Geometry: final body of the model. Coordinates: model frame, mm. Coordinates: 2 decimals unless noted, no trailing zeros. Order: outer loops, then holes, each group sorted by start corner. A loop starts at its lowest first (then second) coordinate and runs counter-clockwise, first axis right, second up. Notation, with made-up numbers: M 47.5,58 L 57.5,58 A14 ccw 57.5,84 Z; hole C -39.5,82.5 d10. An arc over 180 degrees is marked long. Write item = value, one per line. Start each with the question number.
```python
from build123d import *

# Parameters (mm, degrees)
SKETCH_1_R                   = 100
SKETCH_1_R_2                 = 87
SKETCH_1_R_3                 = 2.25
EXTRUDE_1_DEPTH              = 8.5
HOLE_WIZARD_M4_1_D           = 4.8
HOLE_WIZARD_M4_1_CSINK_D     = 9.4
HOLE_WIZARD_M4_1_CSINK_ANGLE = 90


with BuildPart() as part:
    # ｽｹｯﾁ1 → ﾎﾞｽ - 押し出し1 (new body)
    with BuildSketch(Plane.XY):
        Circle(SKETCH_1_R)
        Circle(SKETCH_1_R_2, mode=Mode.SUBTRACT)
        with Locations((0, 93.5)):
            Circle(SKETCH_1_R_3, mode=Mode.SUBTRACT)
        with Locations((93.5, 0)):
            Circle(SKETCH_1_R_3, mode=Mode.SUBTRACT)
        with Locations((0, -93.5)):
            Circle(SKETCH_1_R_3, mode=Mode.SUBTRACT)
        with Locations((-93.5, 0)):
            Circle(SKETCH_1_R_3, mode=Mode.SUBTRACT)
    extrude(amount=EXTRUDE_1_DEPTH)

    # M4 丸皿ねじ用皿穴1 (through all)
    with Locations(Plane.XY.offset(8.5)):
        with Locations((-93.5, 0), (0, 93.5), (93.5, 0), (0, -93.5)):
            CounterSinkHole(HOLE_WIZARD_M4_1_D / 2, HOLE_WIZARD_M4_1_CSINK_D / 2, counter_sink_angle=HOLE_WIZARD_M4_1_CSINK_ANGLE)


solid = part.part
```
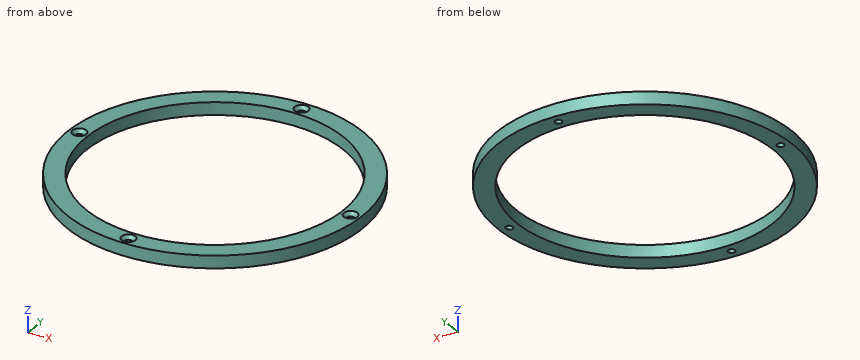
Item 1: Section query C-C on z = 1.75. Output: boundary loops of the cut face in (x, y), and give its area (3 significant figures).
Item 2: First-contact query: pin 1 (3 mm diameter, centred on x = 0, y = -93.5, fed in from -Z); pin 2 (1.5 mm diameter, centred on x = 7, z = 7.5, fed in from -Y); pin 3 (5 mm diameter, centred on y = -33.5, z = 5.5, fed in from -X); pin 4 (4 mm diameter, centred on x = 29, z = 1.5, fed in from -Y). Flat tips, straight axial feed; report the tip coordinate or a pass-through.
Item 3: Material intervals for probe 1 along Y at (x, z) = (0, 3.5); probe 2 along X at (y, z) = (50, 3); probe 3 along Y at (x, z) = (-32, 7.5), sorted ascending. Write a range as [from, to].
Item 4: Section query B-B on y = -60. Output: boundary loops of the cut face in (x, z).
Item 5: Section query A-A on x = 0. Output: boundary loops of the cut face in (y, z), and give its area (3 significant figures).
Ans:
q1.outline = C 0,0 d200; hole C -93.5,0 d4.8; hole C 0,0 d174; hole C 0,-93.5 d4.8; hole C 0,93.5 d4.8; hole C 93.5,0 d4.8
q1.area = 7,560 mm^2
q2.pin_1 = through
q2.pin_2 = -99.8
q2.pin_3 = -95.07
q2.pin_4 = -96.29
q3.probe_1 = [-100, -95.9], [-91.1, -87], [87, 91.1], [95.9, 100]
q3.probe_2 = [-86.6, -71.2], [71.2, 86.6]
q3.probe_3 = [-94.74, -80.9], [80.9, 94.74]
q4.outline = M -80,0 L -63,0 L -63,8.5 L -80,8.5 Z; M 63,0 L 80,0 L 80,8.5 L 63,8.5 Z
q5.outline = M -100,0 L -95.9,0 L -95.9,6.2 L -98.2,8.5 L -100,8.5 Z; M -91.1,0 L -87,0 L -87,8.5 L -88.8,8.5 L -91.1,6.2 Z; M 87,0 L 91.1,0 L 91.1,6.2 L 88.8,8.5 L 87,8.5 Z; M 95.9,0 L 100,0 L 100,8.5 L 98.2,8.5 L 95.9,6.2 Z
q5.area = 129 mm^2
